Could you check a few things on this model? Use its own coordinates, in mm. Face numbers are marked on the shaded views. A direction names the side the tool comes from. Give positions to 0.01 mm unless a question says otherwise; leave off trailing zeros. Loops run counter-clockwise (first coordinate to the right, second up) from the corner with the lowest first, then second, coordinate; pieces in that order, holes last. Notation, with made-up numbers: (-5.75, 22.5) -> (23.25, 22.5) arc R16 cw to (23.25, 45.5) -> close; hole circle Ø9 at (18.5, 30.25). An arc over 180 degrees is marked (long way). Write item = value, one per line. Start each with the question number.
1) I want a section at B-B (x = 7.5). List the corners of the cut face in (y, z) for me.
2) I'm going to push flat-ended pins straight in: pin 1 Ø1.2 at (x, y) = (9.5, 2.5) entering from +Z; pin 2 Ø5 at (x, z) = (0, 0) entering from +Y; pin 3 Ø0.5 at (y, z) = (1, -16) entering from -X. Where does each tip first touch, or does it pass through?
3) If we mould it in two halves opening along X, with no side actions, what happens to the marked faces 1, 2 and 3? For each: +X half, -X half, draft (parallel to the pull), parting line (faces both ways), or undercut.
4) I want a section at C-C (x = 0). List the corners of the cut face in (y, z) for me.
5) I want a section at D-D (y = 1.1). Count the separate pieces of the cut face and the enclosed holes in it, and give its area (3 significant figures).
6) I want a section at A-A (z = -14.5). List the corners of the cut face in (x, y) for me.
7) I need wall thicknesses on probe 1 along X at (y, z) = (3.45, 0); probe 2 along Z at (x, y) = (-10, 1.65); probe 3 along Z at (x, y) = (8, 2.2). Which ranges of each line are inside material? Lowest first, please. Write a range as from..to.
8) On a 3-axis mill with a long thin cutter (end or side, diameter ignored), from which of +Z, -Z, +X, -X, +Y, -Y can I reach the whole of each face in a straight line? I mean the marked faces 4 and 5. Say none if no direction works.
from build123d import *

# Parameters (mm, degrees)
SKETCH1_R           = 2.4
BOSS_EXTRUDE1_DEPTH = 3.9
SKETCH2_R           = 3.05
CUT_EXTRUDE1_DEPTH  = 0.8
SKETCH3_R           = 3.05
CUT_EXTRUDE2_DEPTH  = 0.8


with BuildPart() as part:
    # Sketch1 → Boss-Extrude1 (new body)
    with BuildSketch(Plane(origin=(0, 0, 0), x_dir=(1, 0, 0), z_dir=(0, 1, 0))):
        with BuildLine():
            Line((-7.989922998, 3.65), (4.430077002, 3.65))
            Line((4.430077002, 3.65), (4.430077002, 16.07))
            ThreePointArc((4.430077002, 16.07), (8.080077002, 19.72), (11.730077002, 16.07))
            Line((11.730077002, 16.07), (11.730077002, 0))
            ThreePointArc((11.730077002, 0), (10.661016754, -2.580939751), (8.080077002, -3.65))
            Line((8.080077002, -3.65), (-7.989922998, -3.65))
            ThreePointArc((-7.989922998, -3.65), (-11.639922998, 0), (-7.989922998, 3.65))
        make_face()
        with Locations((0.045077002, 0)):
            Circle(SKETCH1_R, mode=Mode.SUBTRACT)
        with Locations((8.080077002, 8.035)):
            Circle(SKETCH1_R, mode=Mode.SUBTRACT)
        Polygon((8.980077002, 16.97), (10.480077002, 16.97), (10.480077002, 15.17), (8.980077002, 15.17), (8.980077002, 13.67), (7.180077002, 13.67), (7.180077002, 15.17), (5.680077002, 15.17), (5.680077002, 16.97), (7.180077002, 16.97), (7.180077002, 18.47), (8.980077002, 18.47), align=None, mode=Mode.SUBTRACT)
        Polygon((-8.889922998, -2.4), (-7.089922998, -2.4), (-7.089922998, -0.9), (-5.589922998, -0.9), (-5.589922998, 0.9), (-7.089922998, 0.9), (-7.089922998, 2.4), (-8.889922998, 2.4), (-8.889922998, 0.9), (-10.389922998, 0.9), (-10.389922998, -0.9), (-8.889922998, -0.9), align=None, mode=Mode.SUBTRACT)
        Polygon((7.180077002, -2.4), (8.980077002, -2.4), (8.980077002, -0.9), (10.480077002, -0.9), (10.480077002, 0.9), (8.980077002, 0.9), (8.980077002, 2.4), (7.180077002, 2.4), (7.180077002, 0.9), (5.680077002, 0.9), (5.680077002, -0.9), (7.180077002, -0.9), align=None, mode=Mode.SUBTRACT)
    extrude(amount=BOSS_EXTRUDE1_DEPTH)

    # Sketch2 → Cut-Extrude1 (cut)
    with BuildSketch(Plane(origin=(0, 3.9, 0), x_dir=(1, 0, 0), z_dir=(0, 1, 0))):
        Circle(SKETCH2_R)
        with Locations((8.080077002, 8.035)):
            Circle(SKETCH2_R)
    extrude(amount=-CUT_EXTRUDE1_DEPTH, mode=Mode.SUBTRACT)

    # Sketch3 → Cut-Extrude2 (cut)
    with BuildSketch(Plane.XZ):
        with Locations((8.080077002, -8.035)):
            Circle(SKETCH3_R)
        with Locations((0.045077002, 0)):
            Circle(SKETCH3_R)
    extrude(amount=-CUT_EXTRUDE2_DEPTH, mode=Mode.SUBTRACT)


solid = part.part
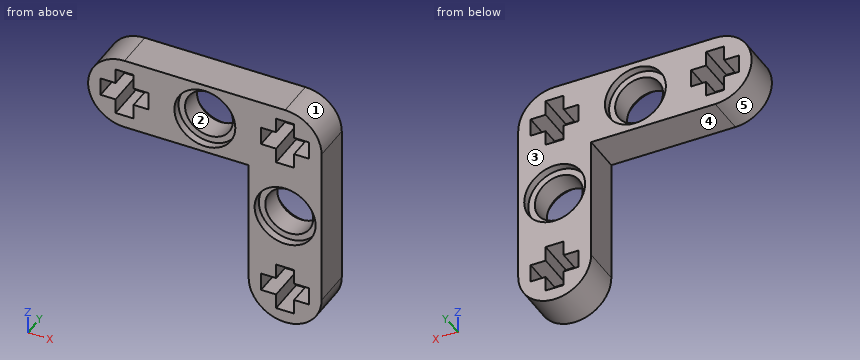
Answer list:
q1.outline = (0, -19.67) -> (3.9, -19.67) -> (3.9, -18.47) -> (0, -18.47) -> close; (0, -13.67) -> (3.9, -13.67) -> (3.9, -11.03) -> (3.1, -11.03) -> (3.1, -10.36) -> (0.8, -10.36) -> (0.8, -11.03) -> (0, -11.03) -> close; (0, -5.04) -> (0.8, -5.04) -> (0.8, -5.71) -> (3.1, -5.71) -> (3.1, -5.04) -> (3.9, -5.04) -> (3.9, -2.4) -> (0, -2.4) -> close; (0, 2.4) -> (3.9, 2.4) -> (3.9, 3.65) -> (0, 3.65) -> close
q2.pin_1 = 3.56
q2.pin_2 = 3.1
q2.pin_3 = 4.43
q3.face_1 = +X half
q3.face_2 = undercut
q3.face_3 = draft
q4.outline = (0, -3.65) -> (3.9, -3.65) -> (3.9, -3.05) -> (3.1, -3.05) -> (3.1, -2.4) -> (0.8, -2.4) -> (0.8, -3.05) -> (0, -3.05) -> close; (0, 3.05) -> (0.8, 3.05) -> (0.8, 2.4) -> (3.1, 2.4) -> (3.1, 3.05) -> (3.9, 3.05) -> (3.9, 3.65) -> (0, 3.65) -> close
q5.separate_pieces = 1
q5.enclosed_holes = 5
q5.area = 195 mm^2
q6.outline = (4.43, 0) -> (7.18, 0) -> (7.18, 3.9) -> (4.43, 3.9) -> close; (8.98, 0) -> (11.73, 0) -> (11.73, 3.9) -> (8.98, 3.9) -> close
q7.probe_1 = -11.64..-10.39, -5.59..-3.05, 3.05..5.68, 10.48..11.73
q7.probe_2 = -3.05..-0.9, 0.9..3.05
q7.probe_3 = -19.72..-18.47, -13.67..-10.43, -5.64..-2.4, 2.4..3.65
q8.face_4 = -Z, -X, +Y, -Y
q8.face_5 = -X, +Y, -Y
